```python
from build123d import *

# Parameters (mm, degrees)
F0_R     = 5.925
F1_DEPTH = 5.9
F3_DEPTH = 12.5


with BuildPart() as f1:
    # F0 (on Top) → F1 (new body)
    with BuildSketch(Plane.XY):
        Circle(F0_R)
    extrude(amount=F1_DEPTH)

    # F2 (on Front) → F3 (cut, symmetric)
    with BuildSketch(Plane.XZ):
        Polygon((-2, 0), (0, 0), (2, 0), (3.819851, 5), (-3.819851, 5), align=None)
    extrude(amount=F3_DEPTH, both=True, mode=Mode.SUBTRACT)


solid = f1.part
```
Part model, mm, in its own coordinate system. Round coordinates to 2 decimals unless told otherwise and drop trailing zeros. Loops run counter-clockwise (first coordinate to the right, second up) from the corner with the lowest first, then second, coordinate; pieces in that order, holes last.
1. Flat gauge pins, fed straight in: pin 1 (1.5 mm diameter, centred on y = -1, z = 3, fed in from -X); pin 2 (3 mm diameter, centred on x = 0, y = -1, fed in from -Z). Where does each tip first touch, or does it go through?
Solutions:
pin 1: stops at x = -5.92
pin 2: stops at z = 5
2. Slice it at B-B (y = -4.75). Give the cut face in (x, z), and give its area (3 significant figures).
Solutions:
outline: (-3.54, 0) - (-2, 0) - (-3.54, 4.24) - close; (-3.54, 5) - (3.54, 5) - (3.54, 5.9) - (-3.54, 5.9) - close; (2, 0) - (3.54, 0) - (3.54, 4.24) - close
area: 12.9 mm2
3. Slice it at C-C (y = 0). Give the cut face in (x, z) (3 decimals).
Solutions:
outline: (-5.925, 0) - (-2, 0) - (-3.82, 5) - (3.82, 5) - (2, 0) - (5.925, 0) - (5.925, 5.9) - (-5.925, 5.9) - close
4. Slice it at A-A (x = -2.25). Give the cut face in (y, z), and give its area (3 significant figures).
Solutions:
outline: (-5.48, 0) - (5.48, 0) - (5.48, 0.69) - (-5.48, 0.69) - close; (-5.48, 5) - (5.48, 5) - (5.48, 5.9) - (-5.48, 5.9) - close
area: 17.4 mm2
5. Slice it at D-D (z = 4.2). Give the cut face in (x, y) (3 decimals).
Solutions:
outline: (-3.529, -4.76) - (-3.529, 4.76) arc R5.925 ccw to start; (3.529, -4.76) arc R5.925 ccw to (3.529, 4.76) - close
6. Drill centre lines: line 1 along Z through (x, y) = (-1, 1); line 2 along X through (y, z) = (4.5, 4.6); line 3 along X through (y, z) = (-2.5, 3.3). Where is each one in solid material? Low to high.
Solutions:
line 1: z = 5 to 5.9
line 2: x = -3.85 to -3.67, 3.67 to 3.85
line 3: x = -5.37 to -3.2, 3.2 to 5.37
7. Two-plate mould, pull along Z, no slides. Class faces 1 (the face through (2.897, -0.078, 2.465)), 2 (the face through (-2.923, -0.078, 2.535)), 3 (the face through (3, 0, 0)), 4 (the face through (0, 0, 5.9)): pulls with the +Z half, pulls with the -Z half, needs draft (parallel to the pull), parting line crosses it, or undercut.
Solutions:
face 1: undercut
face 2: undercut
face 3: pulls with the -Z half
face 4: pulls with the +Z half
